Part model, mm, in its own coordinate system. Face numbers are marked on the shaded views. A direction names the side the tool comes from. Give positions to 0.01 mm unless a question says otherwise; leave off trailing zeros. Write each loop counter-clockwise with the first axis right and the second up, starting at its lowest first coordinate (ties: lowest second). Pieces come first, ordered by that corner, then holes. Notation, with made-up numbers: (-21.5, 23) - (-7.5, 23) arc R12 cw to (-7.5, 33) - close; hole circle Ø1 at (-19.5, -16). An arc over 180 degrees is marked (long way). Answer in a Markdown table with one row per item. Add a question column.
1. Band-saw the part on C-C on z = -6. Write the cut outline in (x, y) (1 decimal), plus the area to 3 significant figures.
2. Band-saw the part on A-A on y = 0. Write the cut outline in (x, z) (3 decimals).
3. Band-saw the part on D-D on z = -8.5. Write the cut outline in (x, y) (1 decimal).
4. Probe line 1 along Y through (x, z) = (0, -3.25); line 2 along Z through (x, y) = (17.5, 7.5) (3 decimals); line 3 along Y through (x, z) = (-10, -8.25). List the from-to ranges inside material, lowest first.
5. Pull direction X, two halves, no side cores. Call the marked faces 1, 2, 3 and 4: released by +X, released by -X, zero draft, split by the parting line, or undercut.
6. Which spindle directions (+Z, -Z, +X, -X, +Y, -Y) get a long thin tool onto all of the face, cutting with end or side? Do the marked faces 5, 6 and 7. Say none if no direction does.
7. Drop flat-ended pins along their axis: pin 1 Ø21.5 at (x, y) = (-0.5, 3) entering from +Z; pin 2 Ø1.5 at (x, z) = (12, -9.5) entering from -Y; pin 3 Ø1.5 at (y, z) = (-10, -8) entering from +X. Give the stop position or say it passes through.
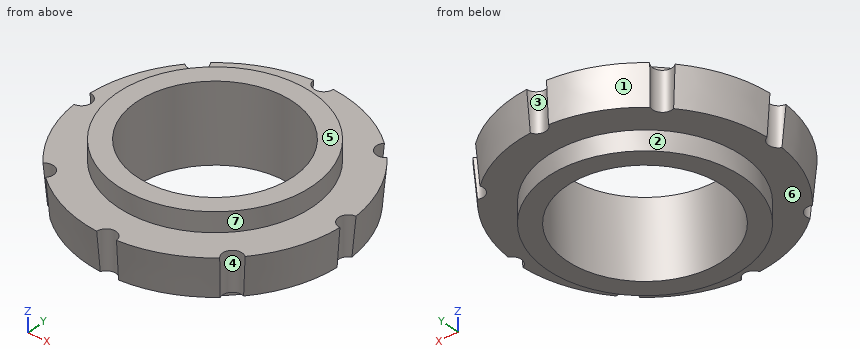
```python
from build123d import *

# Parameters (mm, degrees)
SKETCH2_R         = 1.5875
EXTRUDE1_DEPTH    = 32.728717878
CIRPATTERN1_COUNT = 8


with BuildPart() as part:
    # Sketch1 → Revolve1 (revolve)
    with BuildSketch(Plane(origin=(0, 0, 0), x_dir=(0, 0, -1), z_dir=(1, 0, 0)), mode=Mode.PRIVATE) as revolve1_sk:
        Polygon((0, 15.875), (0, 12.74826), (12.7, 12.74826), (12.7, 15.875), (9.525, 15.875), (9.525, 20.83308), (3.175, 21.40077), (3.175, 15.875), align=None)
    revolve(revolve1_sk.sketch.rotate(Axis((0, 0, 0), (0, 0, -1)), 90), axis=Axis((0, 0, 0), (0, 0, -1)))

    # Sketch2 → Extrude1 (cut, through all)
    with BuildSketch(Plane.XY.offset(-3.175)):
        with Locations((0, 21.40077)):
            Circle(SKETCH2_R)
    extrude1 = extrude(amount=-EXTRUDE1_DEPTH, mode=Mode.SUBTRACT)

    # CirPattern1: Extrude1 ×8 about axis
    cirpattern1_axis = Axis((0, 0, 0), (0, 0, 1))
    for i in range(1, CIRPATTERN1_COUNT):
        add(extrude1.rotate(cirpattern1_axis, i * 360 / CIRPATTERN1_COUNT), mode=Mode.SUBTRACT)


solid = part.part
```
Values:
| question | item | result |
|---|---|---|
| 1 | outline | (-21.1, -1.6) arc R21.1 ccw to (-16, -13.8) arc R1.6 cw to (-13.8, -16) arc R21.1 ccw to (-1.6, -21.1) arc R1.6 cw to (1.6, -21.1) arc R21.1 ccw to (13.8, -16) arc R1.6 cw to (16, -13.8) arc R21.1 ccw to (21.1, -1.6) arc R1.6 cw to (21.1, 1.6) arc R21.1 ccw to (16, 13.8) arc R1.6 cw to (13.8, 16) arc R21.1 ccw to (1.6, 21.1) arc R1.6 cw to (-1.6, 21.1) arc R21.1 ccw to (-13.8, 16) arc R1.6 cw to (-16, 13.8) arc R21.1 ccw to (-21.1, 1.6) arc R1.6 cw to start; hole circle Ø25.5 at (0, 0) |
| 1 | area | 870 mm² |
| 2 | outline | (-19.813, -9.525) - (-15.875, -9.525) - (-15.875, -12.7) - (-12.748, -12.7) - (-12.748, 0) - (-15.875, 0) - (-15.875, -3.175) - (-19.813, -3.175) - close; (12.748, -12.7) - (15.875, -12.7) - (15.875, -9.525) - (19.813, -9.525) - (19.813, -3.175) - (15.875, -3.175) - (15.875, 0) - (12.748, 0) - close |
| 3 | outline | (-20.9, -1.5) arc R20.9 ccw to (-15.8, -13.7) arc R1.6 cw to (-13.7, -15.8) arc R20.9 ccw to (-1.5, -20.9) arc R1.6 cw to (1.5, -20.9) arc R20.9 ccw to (13.7, -15.8) arc R1.6 cw to (15.8, -13.7) arc R20.9 ccw to (20.9, -1.5) arc R1.6 cw to (20.9, 1.5) arc R20.9 ccw to (15.8, 13.7) arc R1.6 cw to (13.7, 15.8) arc R20.9 ccw to (1.5, 20.9) arc R1.6 cw to (-1.5, 20.9) arc R20.9 ccw to (-13.7, 15.8) arc R1.6 cw to (-15.8, 13.7) arc R20.9 ccw to (-20.9, 1.5) arc R1.6 cw to start; hole circle Ø25.5 at (0, 0) |
| 4 | line 1 | y = -19.81 to -12.75, 12.75 to 19.81 |
| 4 | line 2 | z = -9.525 to -3.175 |
| 4 | line 3 | y = -18.41 to -7.91, 7.91 to 18.41 |
| 5 | face 1 | released by -X |
| 5 | face 2 | split by the parting line |
| 5 | face 3 | undercut |
| 5 | face 4 | undercut |
| 6 | face 5 | +Z, +X, -X, +Y, -Y |
| 6 | face 6 | -Z |
| 6 | face 7 | +Z |
| 7 | pin 1 | stops at z = 0 |
| 7 | pin 2 | stops at y = -17.54 |
| 7 | pin 3 | stops at x = 18.83 |
